Input: part model. Units: mm. Frame: model coordinates. Face numbers are marked on the shaded views. A direction names the side the tool comes from. Coordinates: 2 decimals unless noted, no trailing zeros. Order: outer loops, then holes, each group sorted by start corner. A loop starts at its lowest first (then second) coordinate and runs counter-clockwise, first axis right, second up. Notation, with made-up numbers: (29.25, 10) - (49.25, 10) arc R33 cw to (49.25, 46) - close; hole circle Ø4 at (-16, -29). An arc over 180 degrees is marked (long way). One line per question, with ' | ' between items. Start each with the question number.
```python
from build123d import *

# Parameters (mm, degrees)
SKETCH3_R               = 8
BOSS_EXTRUDE1_DEPTH     = 10
BOSS_EXTRUDE2_DEPTH     = 10
CUT_EXTRUDE1_DEPTH      = 34.648922717
CUT_EXTRUDE1_DEPTH_BACK = 34.648922717
SKETCH7_W               = 15.693747285
SKETCH7_H               = 10.5
SKETCH7_W_2             = 16.693747285
SKETCH13_R              = 8.806252715
SKETCH13_R_2            = 4.5
CUT_EXTRUDE2_DEPTH      = 10
FILLET1_R               = 7
CUT_EXTRUDE3_DEPTH      = 10


# Read off the part's stored shape, not the designer's step: Revolve1
with BuildPart() as part:
    # Sketch3 → Boss-Extrude1 (new, symmetric)
    with BuildSketch(Plane(origin=(0, 0, 0), x_dir=(1, 0, 0), z_dir=(0, 1, 0))):
        with Locations(Location((0, 0, 0), (0, 0, 270))):
            Circle(SKETCH3_R)
    extrude(amount=BOSS_EXTRUDE1_DEPTH, both=True)

    # Sketch6 → Boss-Extrude2 (add, symmetric)
    with BuildSketch(Plane(origin=(0, 0, 0), x_dir=(1, 0, 0), z_dir=(0, 1, 0))):
        with BuildLine():
            Line((7.193747285, -3.5), (14.806252715, -3.5))
            Line((14.806252715, -3.5), (22, -8))
            ThreePointArc((22, -8), (30, 0), (22, 8))
            Line((22, 8), (14.806252715, 3.5))
            Line((14.806252715, 3.5), (7.193747285, 3.5))
            ThreePointArc((7.193747285, 3.5), (8, 0), (7.193747285, -3.5))
        make_face()
    extrude(amount=BOSS_EXTRUDE2_DEPTH, both=True)

    # Sketch7 → Cut-Extrude1 (cut, two sides: drawn at the far end of the back side and taken through both)
    with BuildSketch(Plane.XY.offset(3.5).offset(-CUT_EXTRUDE1_DEPTH_BACK)):
        with Locations((-0.653126357, -5.25)):
            Rectangle(SKETCH7_W, SKETCH7_H)
        with Locations((22.153126358, 5.25)):
            Rectangle(SKETCH7_W_2, SKETCH7_H)
    extrude(amount=CUT_EXTRUDE1_DEPTH + CUT_EXTRUDE1_DEPTH_BACK, mode=Mode.SUBTRACT)

    # Sketch8 → Cut-Revolve2 (revolve, cut)
    with BuildSketch(Plane.XY, mode=Mode.PRIVATE) as cut_revolve2_sk:
        Polygon((0, 10), (0, 0), (3, 0), (3, 6), (5, 8), (5, 10), align=None)
    revolve(cut_revolve2_sk.sketch.rotate(Axis((0, 11.592954006, 0), (0, -1, 0)), 90), axis=Axis((0, 11.592954006, 0), (0, -1, 0)), mode=Mode.SUBTRACT)

    # Revolve1 outline → Revolve1 (revolve)
    with BuildSketch(Plane(origin=(22, 0, 0), x_dir=(1, 0, 0), z_dir=(0, 0, 1))):
        Polygon((0, 10), (0, 0), (2.5, 0), (2.5, 6.207106781), (4.5, 8.207106781), (4.5, 10), align=None)
    revolve(axis=Axis((22, 0, 0), (0, 1, 0)))

    # Sketch13 → Cut-Extrude2 (cut)
    with BuildSketch(Plane(origin=(0, 10, 0), x_dir=(1, 0, 0), z_dir=(0, 1, 0))):
        with Locations((22, 0)):
            Circle(SKETCH13_R)
        with Locations(Location((22, 0, 0), (0, 0, 270))):
            Circle(SKETCH13_R_2, mode=Mode.SUBTRACT)
    extrude(amount=-CUT_EXTRUDE2_DEPTH, mode=Mode.SUBTRACT)

    # Fillet1
    fillet1_edges = [part.edges().sort_by_distance(p)[0] for p in [
        (22, -5, -8),
        (22, -5, 8),
    ]]
    fillet(fillet1_edges, radius=FILLET1_R)

    # Sketch14 → Cut-Extrude3 (cut)
    with BuildSketch(Plane.XZ.offset(10)):
        with BuildLine():
            Line((8.693747285, -3.5), (8.693747285, 0.353821083))
            ThreePointArc((8.693747285, 0.353821083), (6.057708316, 6.717782114), (-0.306252715, 9.353821083))
            Line((-0.306252715, 9.353821083), (-1.238376204, 9.353821083))
            ThreePointArc((-1.238376204, 9.353821083), (-36.061646902, -27.818232152), (8.693747285, -3.5))
        make_face()
    extrude(amount=-CUT_EXTRUDE3_DEPTH, mode=Mode.SUBTRACT)


solid = part.part
```
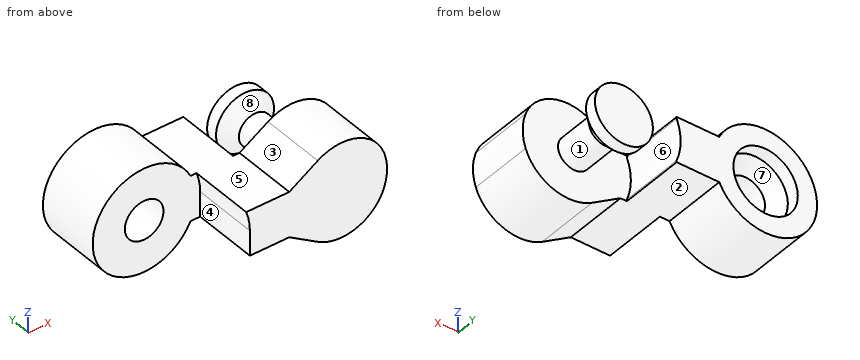
(1) Material intervals for line 1 along Y through (x, z) = (-2.5, 6.75); line 2 along Z through (x, y) = (11.5, -6); line 3 along Y through (x, z) = (20.5, 5.25), sorted ascending. Write a range as from..to.
(2) Draft query along Y for the marked faces 6, 7 and 8. Return one class per face: +Y half, -Y half, draft (parallel to the pull), parting line (faces both ways), or undercut.
(3) Section D-D (y = -3.75). Output: boundary loops of the cut face in (x, z).
(4) Section C-C (z = 5.75). Output: boundary loops of the cut face in (x, y).
(5) Pin query (flat end, axial travel): pin 1 (1 mm diameter, centred on x = 21, y = -0.5, fed in from -Z); pin 2 (4 mm diameter, centred on x = 13, y = -0.5, fed in from +Z); pin 3 (4 mm diameter, centred on x = 15, y = -5, fed in from +Z); pin 4 (7.5 mm diameter, centred on x = 25.5, z = 3, fed in from +Y). Return the tip coordinate at first contact, or that it passes through.
(6) Section A-A (x = 0). Output: boundary loops of the cut face in (y, z).
(7) Section B-B (y = 0.75). Output: boundary loops of the cut face in (x, z).
(8) Reachability of the marked faces 1, 2, 3, 4 and 5 from +Z, -Z, +X, -X, +Y, -Y: full face, straight path, thin tool, end or side. Return the list, or none.
Worked answers:
1) line 1: y = 0..10 | line 2: z = -3.5..3.5 | line 3: y = -10..0
2) face 6: draft | face 7: +Y half | face 8: undercut
3) outline: (8.13, 3.5) arc R9 cw to (8.69, 0.35) - (8.69, -3.5) - (14.81, -3.5) - (19.23, -6.27) arc R7 ccw to (29.54, -2.66) arc R8 ccw to (29.54, 2.66) arc R7 ccw to (19.23, 6.27) - (14.81, 3.5) - close
4) outline: (-5.56, 0) - (5.56, 0) - (5.56, 10) - (-5.56, 10) - close; (18.4, -10) - (27.38, -10) - (27.38, 0) - (18.4, 0) - close
5) pin 1: stops at z = -7.18 | pin 2: stops at z = 3.62 | pin 3: stops at z = 4.87 | pin 4: stops at y = 10
6) outline: (0, -8) - (10, -8) - (10, -5) - (8, -5) - (6, -3) - (0, -3) - close; (0, 3) - (6, 3) - (8, 5) - (10, 5) - (10, 8) - (0, 8) - close
7) outline: (7.19, -3.5) - (13.81, -3.5) - (13.81, -3.23) arc R8.81 cw to (13.81, 3.23) - (13.81, 3.5) - (7.19, 3.5) arc R8 ccw (long way) to start; circle Ø5 at (22, 0); hole circle Ø6 at (0, 0)
8) face 1: none | face 2: -Z, +Y, -Y | face 3: +Z, -X, +Y, -Y | face 4: -Z, -X, -Y | face 5: +Z, +Y, -Y
